from build123d import *

# Parameters (mm, degrees)
F0_R     = 25.142108
F1_DEPTH = 2
F2_R     = 18.693726
F3_DEPTH = 10
F5_DEPTH = 50


with BuildPart() as f1:
    # F0 (on Front) → F1 (new body)
    with BuildSketch(Plane.XZ):
        Circle(F0_R)
    extrude(amount=F1_DEPTH)

    # F2 (on face) → F3 (join)
    with BuildSketch(Plane.XZ.offset(2)):
        Circle(F2_R)
    extrude(amount=F3_DEPTH)

    # F4 (on face) → F5 (join)
    with BuildSketch(Plane.XZ.offset(12)):
        Polygon((-12.644799, -5.127543), (-3.875029, -13.083073), (7.812717, -11.186782), (13.617328, -0.866616), (9.167813, 10.106129), (-2.185252, 13.468753), (-11.892778, 6.689131), align=None)
    extrude(amount=F5_DEPTH)


solid = f1.part
Read the model definition and answer for the solid it produces. Units are mm, in the model's axes. A direction names the side the tool comes from. Give positions to 0.01 mm unless a question says otherwise; leave off trailing zeros. Write each loop counter-clockwise with the first axis right and the second up, starting at its lowest first coordinate (ties: lowest second). Pieces come first, ordered by that corner, then holes. Notation, with made-up numbers: (15, -29) - (32, -29) arc R21 cw to (32, -1) - close; hole circle Ø9 at (-36.75, 46). An arc over 180 degrees is marked (long way). Return JSON: item names as keys, results as strings.
Q1. A cutting plane is placed at B-B, the plane x = 0. Determine the outline of the cut face in (y, z), and give its area (3 significant figures).
Reply:
{"outline": "(-62, -12.45) - (-12, -12.45) - (-12, -18.69) - (-2, -18.69) - (-2, -25.14) - (0, -25.14) - (0, 25.14) - (-2, 25.14) - (-2, 18.69) - (-12, 18.69) - (-12, 12.82) - (-62, 12.82) - close", "area": "1,740 mm²"}
Q2. Given P1, Ø12, axis at x = 18, y = -44, coming from the -Z side; P2, Ø10, axis at x = 7.5, z = -7.5, coming from the +Y side; P3, Ø5, axis at y = -13, z = 1, coming from the -X side; P4, Ø6, axis at y = -24.5, z = -16, coming from the -X side, each flat-ended and moving along its own axis, determine where each tip first touches the part or whether it passes through.
Reply:
{"P1": "z = -3.74", "P2": "y = 0", "P3": "x = -18.69", "P4": "x = -3.97"}
Q3. For faces 1 (the face through (12.2, -12, -3.9)), 2 (the face through (10.674, -36.65, -6.099)), 3 (the face through (3.571, -36.65, 11.764)), determine the directions among +Z, -Z, +X, -X, +Y, -Y from which every point of the face is accessible in a straight line to the end or side of a thin tool.
Reply:
{"face 1": "-Y", "face 2": "-Z, +X, -Y", "face 3": "+Z, +X, -Y"}
Q4. Consider line 1 along Y through (x, z) = (-19, 6); line 2 along Y through (x, z) = (7.5, -16); line 3 along Z through (x, y) = (-10.5, -53). Determine where each line is inside the solid, lowest interval first. Write a range as [from, to].
Reply:
{"line 1": "[-2, 0]", "line 2": "[-12, 0]", "line 3": "[-7.07, 7.66]"}
Q5. A cutting plane is placed at A-A, the plane y = -40.5. Determine the outline of the cut face in (x, z), and give its area (3 significant figures).
Reply:
{"outline": "(-12.64, -5.13) - (-3.88, -13.08) - (7.81, -11.19) - (13.62, -0.87) - (9.17, 10.11) - (-2.19, 13.47) - (-11.89, 6.69) - close", "area": "509 mm²"}
Q6. A cutting plane is placed at C-C, the plane z = 16. Determine the outline of the cut face in (x, y), and give its area (3 significant figures).
Reply:
{"outline": "(-19.39, -2) - (-9.67, -2) - (-9.67, -12) - (9.67, -12) - (9.67, -2) - (19.39, -2) - (19.39, 0) - (-19.39, 0) - close", "area": "271 mm²"}
Q7. A cutting plane is placed at D-D, the plane x = 6. Determine the outline of the cut face in (y, z).
Reply:
{"outline": "(-62, -11.48) - (-12, -11.48) - (-12, -17.7) - (-2, -17.7) - (-2, -24.42) - (0, -24.42) - (0, 24.42) - (-2, 24.42) - (-2, 17.7) - (-12, 17.7) - (-12, 11.04) - (-62, 11.04) - close"}
